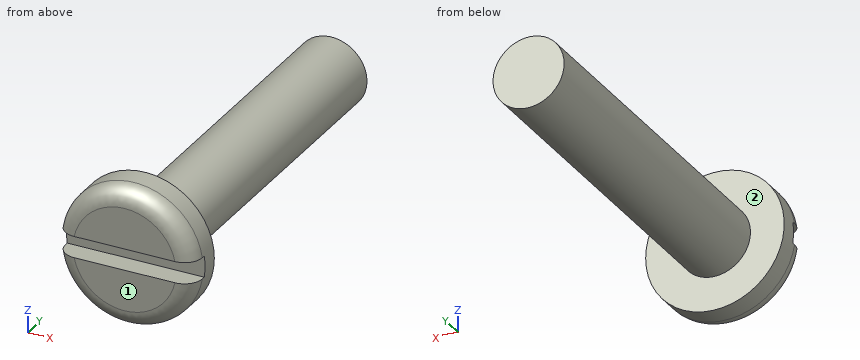
from build123d import *

# Parameters (mm, degrees)
F0_R     = 3.9
F1_DEPTH = 2.2
F2_R     = 1
F3_W     = 8
F3_H     = 1.2
F4_DEPTH = 1.2
F5_R     = 2
F6_DEPTH = 20


with BuildPart() as f1:
    # F0 (on Front) → F1 (new body)
    with BuildSketch(Plane.XZ):
        Circle(F0_R)
    extrude(amount=-F1_DEPTH)

    # F2
    f2_edges = [f1.edges().sort_by_distance(p)[0] for p in [
        (-3.9, 0, 0),
    ]]
    fillet(f2_edges, radius=F2_R)

    # F3 (on face) → F4 (cut)
    with BuildSketch(Plane.XZ):
        Rectangle(F3_W, F3_H)
    extrude(amount=-F4_DEPTH, mode=Mode.SUBTRACT)

    # F5 (on face) → F6 (join)
    with BuildSketch(Plane(origin=(0, 2.2, 0), x_dir=(-1, 0, 0), z_dir=(0, 1, 0))):
        Circle(F5_R)
    extrude(amount=F6_DEPTH)


solid = f1.part
Model file for the job. Use its own axes, mm. Face numbers are marked on the shaded views. A direction names the side the tool comes from. Round coordinates to 2 decimals unless told otherwise and drop trailing zeros. Loops run counter-clockwise (first coordinate to the right, second up) from the corner with the lowest first, then second, coordinate; pieces in that order, holes last.
1. Drop flat-ended pins along their axis: P1, Ø0.6, axis at x = 1.5, y = 0.5, coming from the +Z side; P2, Ø3, axis at y = 14.5, z = -0.5, coming from the -X side; P3, Ø0.6, axis at x = 1, y = 0.5, coming from the -Z side. Give the stop position or say it passes through.
Check values:
P1: stops at z = 3.64
P2: stops at x = -2
P3: stops at z = -3.78
2. Tool access for the marked faces 1 and 2: list every direction of +Z, -Z, +X, -X, +Y, -Y with a clear straight run to the whole face (end or side of a thin tool).
Check values:
face 1: +Z, -Z, +X, -X, -Y
face 2: +Y
3. Band-saw the part on C-C, the plane y = 9.5. List the corners of the cut face in (x, z).
Check values:
outline: circle Ø4 at (0, 0)
4. Band-saw the part on A-A, the plane x = 0. List the corners of the cut face in (y, z).
Check values:
outline: (0, -2.9) arc R1 ccw to (1, -3.9) - (2.2, -3.9) - (2.2, -2) - (22.2, -2) - (22.2, 2) - (2.2, 2) - (2.2, 3.9) - (1, 3.9) arc R1 ccw to (0, 2.9) - (0, 0.6) - (1.2, 0.6) - (1.2, -0.6) - (0, -0.6) - close
5. Wall check: probe 1 along Y at (x, z) = (-2.5, 0.5); probe 2 along Y at (x, z) = (-2.5, -1.5); probe 3 along X at (y, z) = (3.5, 1.25). Give the ranges that are in metal, low to high.
Check values:
probe 1: y = 1.2 to 2.2
probe 2: y = 0 to 2.2
probe 3: x = -1.56 to 1.56
6. Band-saw the part on B-B, the plane z = 0. List the corners of the cut face in (x, y).
Check values:
outline: (-3.9, 1.2) - (3.9, 1.2) - (3.9, 2.2) - (2, 2.2) - (2, 22.2) - (-2, 22.2) - (-2, 2.2) - (-3.9, 2.2) - close
